```python
from build123d import *

# Parameters (mm, degrees)
F0_W     = 18.75
F0_H     = 33.2
F0_R     = 1.5
F1_DEPTH = 3


with BuildPart() as f1:
    # F0 (on Top) → F1 (new body)
    with BuildSketch(Plane.XY):
        Rectangle(F0_W, F0_H)
        with BuildLine():
            Line((-6.375, -11.6), (-6.375, 11.6))
            Line((-6.375, 11.6), (6.375, 11.6))
            Line((6.375, 11.6), (6.375, -11.6))
            Line((6.375, -11.6), (4, -11.6))
            Line((4, -11.6), (4, -14.1))
            Line((4, -14.1), (1.414214, -14.1))
            ThreePointArc((1.414214, -14.1), (0, -15.1), (-1.414214, -14.1))
            Line((-1.414214, -14.1), (-4, -14.1))
            Line((-4, -14.1), (-4, -11.6))
            Line((-4, -11.6), (-6.375, -11.6))
        make_face(mode=Mode.SUBTRACT)
        with Locations((0, 13.6)):
            Circle(F0_R, mode=Mode.SUBTRACT)
    extrude(amount=F1_DEPTH)


solid = f1.part
```
Input: part model. Units: mm. Frame: model coordinates. A direction names the side the tool comes from. Give positions to 0.01 mm unless a question says otherwise; leave off trailing zeros. Order: outer loops, then holes, each group sorted by start corner. A loop starts at its lowest first (then second) coordinate and runs counter-clockwise, first axis right, second up. Notation, with made-up numbers: M 28.5,39.5 L 33.5,39.5 A23 ccw 33.5,60.5 Z; hole C -33.5,34 d4. An arc over 180 degrees is marked long. Return JSON: item names as keys, results as strings.
1) Section query D-D on x = 0. Output: boundary loops of the cut face in (y, z).
Taken from the geometry:
{"outline": "M -16.6,0 L -15.1,0 L -15.1,3 L -16.6,3 Z; M 11.6,0 L 12.1,0 L 12.1,3 L 11.6,3 Z; M 15.1,0 L 16.6,0 L 16.6,3 L 15.1,3 Z"}
2) Section query B-B on x = 3. Output: boundary loops of the cut face in (y, z).
Taken from the geometry:
{"outline": "M -16.6,0 L -14.1,0 L -14.1,3 L -16.6,3 Z; M 11.6,0 L 16.6,0 L 16.6,3 L 11.6,3 Z"}
3) Section query C-C on z = 1. Output: boundary loops of the cut face in (x, y) (3 decimals), and give its area (3 significant figures).
Taken from the geometry:
{"outline": "M -9.375,-16.6 L 9.375,-16.6 L 9.375,16.6 L -9.375,16.6 Z; hole M -6.375,-11.6 L -4,-11.6 L -4,-14.1 L -1.414,-14.1 A1.5 ccw 1.414,-14.1 L 4,-14.1 L 4,-11.6 L 6.375,-11.6 L 6.375,11.6 L -6.375,11.6 Z; hole C 0,13.6 d3", "area": "298 mm2"}
4) Access query for faces 4 (the face through (-9.375, 0, 1)), 5 (the face through (4, -13, 1)). Directions: +Z, -Z, +X, -X, +Y, -Y. A direction counts if a zero-diameter tool reaches every point of the face in a straight line with its end or side. Return the directions, or none.
Taken from the geometry:
{"face 4": "+Z, -Z, -X, +Y, -Y", "face 5": "+Z, -Z"}
5) Section query A-A on y = 0. Output: boundary loops of the cut face in (x, z) (3 decimals), and give its area (3 significant figures).
Taken from the geometry:
{"outline": "M -9.375,0 L -6.375,0 L -6.375,3 L -9.375,3 Z; M 6.375,0 L 9.375,0 L 9.375,3 L 6.375,3 Z", "area": "18.0 mm2"}
6) Mould query, pull axis X, two halves, no side actions, for faces 1 (the face through (9.375, 0, 1)), 2 (the face through (0, 11.6, 1)), 3 (the face through (0, 16.6, 1)). Classes: released by +X, released by -X, zero draft, split by the parting line, or undercut.
Taken from the geometry:
{"face 1": "released by +X", "face 2": "undercut", "face 3": "zero draft"}
7) Line query: L1, parallel to Y at x = 0, z = 1.45; L2, parallel to Y at x = -4.5, z = 2.85; L3, parallel to X at y = -11, z = 0.8 (3 decimals). Output: solid intervals per line, ascending. Write a range as [from, to].
Taken from the geometry:
{"L1": "y = [-16.6, -15.1], [11.6, 12.1], [15.1, 16.6]", "L2": "y = [-16.6, -11.6], [11.6, 16.6]", "L3": "x = [-9.375, -6.375], [6.375, 9.375]"}
